from build123d import *

# Parameters (mm, degrees)
BOSS_EXTRUDE1_DEPTH = 3.175
SKETCH2_R           = 2.1
CUT_EXTRUDE1_DEPTH  = 243.144751389
SKETCH3_R           = 2.1
CUT_EXTRUDE2_DEPTH  = 10
SKETCH4_R           = 2.1
CUT_EXTRUDE3_DEPTH  = 243.144751389


with BuildPart() as part:
    # Sketch1 → Boss-Extrude1 (new body)
    with BuildSketch(Plane.YZ):
        with BuildLine():
            Line((-208, 32), (208, 32))
            ThreePointArc((208, 32), (240, 0), (208, -32))
            Line((208, -32), (-208, -32))
            ThreePointArc((-208, -32), (-240, 0), (-208, 32))
        make_face()
    extrude(amount=BOSS_EXTRUDE1_DEPTH)

    # Sketch2 → Cut-Extrude1 (cut, through all)
    with BuildSketch(Plane.YZ.offset(3.175)):
        with Locations(Location((208, 12, 0), (0, 0, 270))):
            Circle(SKETCH2_R)
        with Locations(Location((218.392304845, 6, 0), (0, 0, 270))):
            Circle(SKETCH2_R)
        with Locations(Location((218.392304845, -6, 0), (0, 0, 270))):
            Circle(SKETCH2_R)
        with Locations(Location((208, -12, 0), (0, 0, 270))):
            Circle(SKETCH2_R)
        with Locations(Location((197.607695155, -6, 0), (0, 0, 270))):
            Circle(SKETCH2_R)
        with Locations(Location((197.607695155, 6, 0), (0, 0, 270))):
            Circle(SKETCH2_R)
    extrude(amount=-CUT_EXTRUDE1_DEPTH, mode=Mode.SUBTRACT)

    # Sketch3 → Cut-Extrude2 (cut)
    with BuildSketch(Plane.YZ.offset(3.175)):
        with Locations(Location((-208, -12, 0), (0, 0, 270))):
            Circle(SKETCH3_R)
        with Locations(Location((-197.607695155, -6, 0), (0, 0, 270))):
            Circle(SKETCH3_R)
        with Locations(Location((-197.607695155, 6, 0), (0, 0, 270))):
            Circle(SKETCH3_R)
        with Locations(Location((-208, 12, 0), (0, 0, 270))):
            Circle(SKETCH3_R)
        with Locations(Location((-218.392304845, 6, 0), (0, 0, 270))):
            Circle(SKETCH3_R)
        with Locations(Location((-218.392304845, -6, 0), (0, 0, 270))):
            Circle(SKETCH3_R)
    extrude(amount=-CUT_EXTRUDE2_DEPTH, mode=Mode.SUBTRACT)

    # Sketch4 → Cut-Extrude3 (cut, through all)
    with BuildSketch(Plane.YZ.offset(3.175)):
        with Locations(Location((-208, 12, 0), (0, 0, 270))):
            Circle(SKETCH4_R)
        with Locations(Location((-208, 28, 0), (0, 0, 270))):
            Circle(SKETCH4_R)
        with Locations(Location((-208, -28, 0), (0, 0, 90))):
            Circle(SKETCH4_R)
        with Locations(Location((-176, 28, 0), (0, 0, 270))):
            Circle(SKETCH4_R)
        with Locations(Location((-176, -28, 0), (0, 0, 90))):
            Circle(SKETCH4_R)
        with Locations(Location((-144, 28, 0), (0, 0, 270))):
            Circle(SKETCH4_R)
        with Locations(Location((-144, -28, 0), (0, 0, 90))):
            Circle(SKETCH4_R)
        with Locations(Location((-112, 28, 0), (0, 0, 270))):
            Circle(SKETCH4_R)
        with Locations(Location((-112, -28, 0), (0, 0, 90))):
            Circle(SKETCH4_R)
        with Locations(Location((-80, 28, 0), (0, 0, 270))):
            Circle(SKETCH4_R)
        with Locations(Location((-80, -28, 0), (0, 0, 90))):
            Circle(SKETCH4_R)
        with Locations(Location((-48, 28, 0), (0, 0, 270))):
            Circle(SKETCH4_R)
        with Locations(Location((-48, -28, 0), (0, 0, 90))):
            Circle(SKETCH4_R)
        with Locations(Location((-16, 28, 0), (0, 0, 270))):
            Circle(SKETCH4_R)
        with Locations(Location((-16, -28, 0), (0, 0, 90))):
            Circle(SKETCH4_R)
        with Locations(Location((16, 28, 0), (0, 0, 270))):
            Circle(SKETCH4_R)
        with Locations(Location((16, -28, 0), (0, 0, 90))):
            Circle(SKETCH4_R)
        with Locations(Location((48, 28, 0), (0, 0, 270))):
            Circle(SKETCH4_R)
        with Locations(Location((48, -28, 0), (0, 0, 90))):
            Circle(SKETCH4_R)
        with Locations(Location((80, 28, 0), (0, 0, 270))):
            Circle(SKETCH4_R)
        with Locations(Location((80, -28, 0), (0, 0, 90))):
            Circle(SKETCH4_R)
        with Locations(Location((112, 28, 0), (0, 0, 270))):
            Circle(SKETCH4_R)
        with Locations(Location((112, -28, 0), (0, 0, 90))):
            Circle(SKETCH4_R)
        with Locations(Location((144, 28, 0), (0, 0, 270))):
            Circle(SKETCH4_R)
        with Locations(Location((144, -28, 0), (0, 0, 90))):
            Circle(SKETCH4_R)
        with Locations(Location((176, 28, 0), (0, 0, 270))):
            Circle(SKETCH4_R)
        with Locations(Location((176, -28, 0), (0, 0, 90))):
            Circle(SKETCH4_R)
        with Locations(Location((208, 28, 0), (0, 0, 270))):
            Circle(SKETCH4_R)
        with Locations(Location((208, -28, 0), (0, 0, 90))):
            Circle(SKETCH4_R)
    extrude(amount=-CUT_EXTRUDE3_DEPTH, mode=Mode.SUBTRACT)


solid = part.part
Geometry check sheet. Reference: the model listing, model coordinates, mm. Give positions to 0.01 mm unless a question says otherwise; leave off trailing zeros.
1. Sectioned sample at A-A (x = 1.9). State how many separate pieces and enclosed holes the cut face has, then the cut area to 3 significant figures.
Completed:
separate pieces: 1
enclosed holes: 40
area: 29,300 mm2
2. Depth check by flat-ended pin: pin 1 (1 mm diameter, centred on x = 0.5, z = -23.5, fed in from +Y). Enter the tip coordinate at first touch or a pass-through.
Completed:
pin 1: stops at y = 230.25
3. Scan lines: line 1 (Z direction, x = 0.5, y = 144); line 2 (Z direction, x = 1.1, y = -208); line 3 (Z direction, x = 1.6, y = -79). Record each from-to range of solid material in increasing order.
Completed:
line 1: z = -32 to -30.1, -25.9 to 25.9, 30.1 to 32
line 2: z = -32 to -30.1, -25.9 to -14.1, -9.9 to 9.9, 14.1 to 25.9, 30.1 to 32
line 3: z = -32 to -29.85, -26.15 to 26.15, 29.85 to 32
